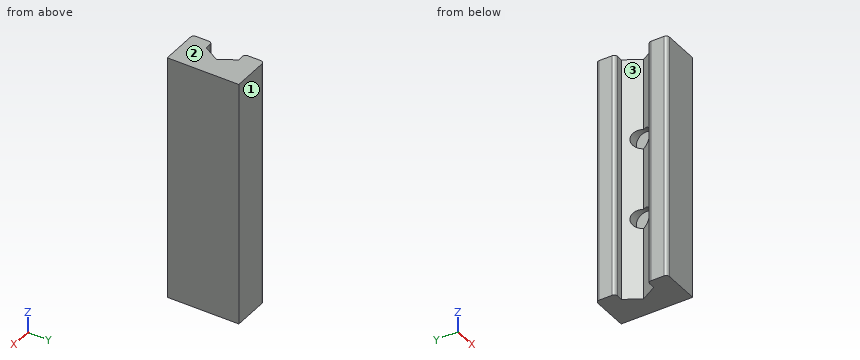
```python
from build123d import *

# Parameters (mm, degrees)
F1_DEPTH = 38.1
F3_START = -2.54
F2_R     = 1.54305
F3_DEPTH = 1.524
F4_R     = 0.508


with BuildPart() as f1:
    # F0 (on Top) → F1 (new body)
    with BuildSketch(Plane.XY):
        Polygon((-31.75, 8.0264), (-34.7726, 8.0264), (-34.7726, 4.9911), (-33.3281273615, 4.9911), (-31.883654723, 2.4892), (-33.3281273615, -0.0127), (-34.7726, -0.0127), (-34.7726, -3.048), (-31.75, -3.048), (-28.702, -3.048), (-28.702, 8.0264), align=None)
    extrude(amount=F1_DEPTH)

    # F2 (on face) → F3 (cut)
    with BuildSketch(Plane.YZ.offset(-28.702).offset(F3_START)):
        with Locations((2.4892, 25.4)):
            Circle(F2_R)
        with Locations((2.4892, 12.7)):
            Circle(F2_R)
    extrude(amount=-F3_DEPTH, mode=Mode.SUBTRACT)

    # F4
    f4_edges = [f1.edges().sort_by_distance(p)[0] for p in [
        (-34.7726, -3.048, 19.05),
        (-34.7726, 8.0264, 19.05),
        (-34.7726, 4.9911, 19.05),
        (-34.7726, -0.0127, 19.05),
    ]]
    fillet(f4_edges, radius=F4_R)


solid = f1.part
```
Geometry: final body of the model. Coordinates: model frame, mm. Face numbers are marked on the shaded views. Coordinates: 2 decimals unless noted, no trailing zeros. Loops run counter-clockwise (first coordinate to the right, second up) from the corner with the lowest first, then second, coordinate; pieces in that order, holes last. Notation, with made-up numbers: M 20.25,85.5 L 47.25,85.5 A29 ccw 47.25,119.5 Z; hole C -22.5,87 d9. An arc over 180 degrees is marked long. Put each result on its own line as item: value.
(1) Material intervals for probe 1 along Y at (x, z) = (-32.3, 12.7); probe 2 along Z at (x, y) = (-31.5, 2); probe 3 along Y at (x, z) = (-32, 27), sorted ascending.
Answer sheet:
probe 1: y = -3.05 to 0.95, 4.03 to 8.03
probe 2: z = 0 to 11.24, 14.16 to 23.94, 26.86 to 38.1
probe 3: y = -3.05 to 2.29, 2.69 to 8.03
(2) First-contact query: pin 1 (3.5 mm diameter, centred on y = 2, z = 12, fed in from -X). Flat tip, straight axial feed; report the tip coordinate or a pass-through.
Answer sheet:
pin 1: stops at x = -33.18
(3) Cut plane A-A on z = 30.5. Return the cut outline in (x, y), then the cut area to 3 significant figures.
Answer sheet:
outline: M -34.77,-2.54 A0.51 ccw -34.26,-3.05 L -28.7,-3.05 L -28.7,8.03 L -34.26,8.03 A0.51 ccw -34.77,7.52 L -34.77,5.5 A0.51 ccw -34.26,4.99 L -33.33,4.99 L -31.88,2.49 L -33.33,-0.01 L -34.26,-0.01 A0.51 ccw -34.77,-0.52 Z
area: 56.2 mm^2
(4) Draft query along Y for the marked faces 1, 2 and 3. Return one class per face: pulls with the +Y half, pulls with the -Y half, needs draft (parallel to the pull), parting line crosses it, or undercut.
Answer sheet:
face 1: pulls with the +Y half
face 2: needs draft
face 3: undercut
